Geometry: see drawing. Coordinates: mm, zero at the bounding-box minimum. A direction names the side the tool comes from. Give positions to 0.01 mm unless a question says otherwise; leave off trailing zeros. Order: outer loops, then holes, each group sorted by start corner. A loop starts at its lowest first (then second) coordinate and runs counter-clockwise, first axis right, second up. Notation, with made-up numbers: (20.25, 31) - (73.25, 31) arc R31 ccw to (73.25, 64) - close; hole circle Ø2 at (-13.75, 24). An arc over 180 degrees is marked (long way). One line per question, with ' | ' between items. Start each with the question number.
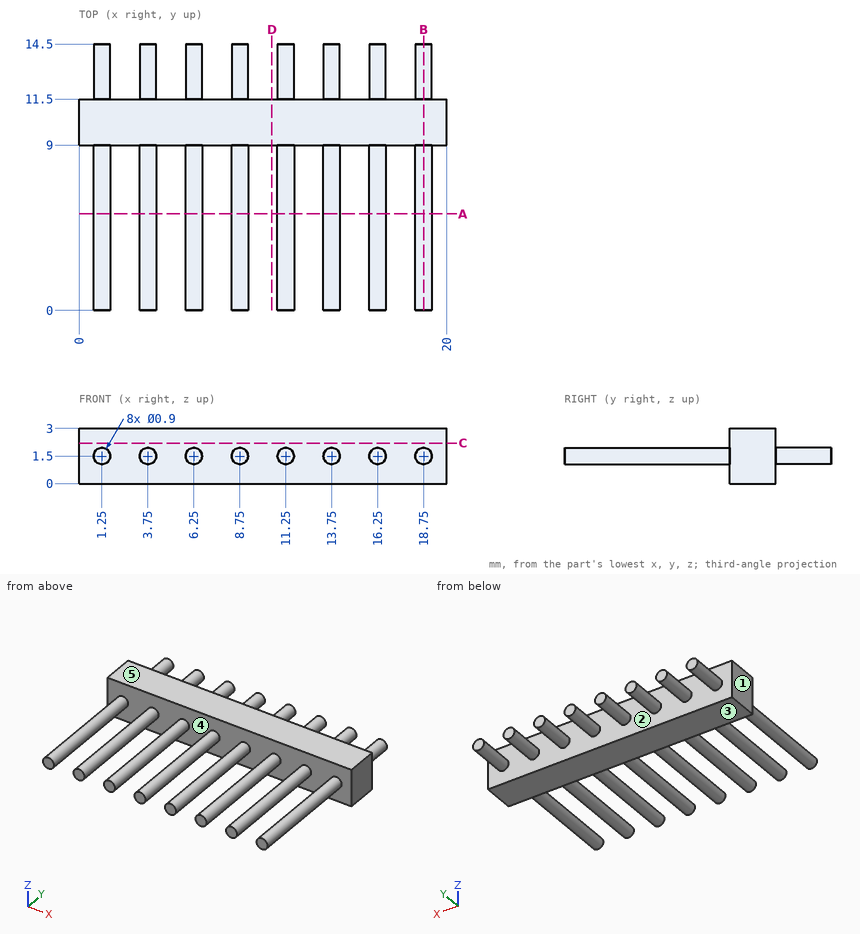
(1) Cut plane A-A, the plane y = 5.25. Return the cut outline in (x, z).
(2) Pull-direction query (X, two-part tool) for the marked faces 1, 2 and 3; classes: +X half, -X half, draft (parallel to the pull), parting line (faces both ways), or undercut.
(3) Cut plane B-B, the plane x = 18.75. Return the cut outline in (y, z).
(4) Material intervals for line 1 along Y through (x, z) = (14.75, 0.9); line 2 along Z through (x, y) = (13.5, 6.5), sorted ascending. Write a range as from..to.
(5) Cut plane C-C, the plane z = 2.2. Return the cut outline in (x, y), plus the area to 3 significant figures.
(6) Access query for the marked faces 4 and 5. Directions: +Z, -Z, +X, -X, +Y, -Y. A direction counts if a zero-diameter tool reaches every point of the face in a straight line with its end or side. Return the directions, or none.
(7) Cut plane D-D, the plane x = 10.5. Return the cut outline in (y, z).
Results are:
1) outline: circle Ø0.9 at (1.25, 1.5); circle Ø0.9 at (3.75, 1.5); circle Ø0.9 at (6.25, 1.5); circle Ø0.9 at (8.75, 1.5); circle Ø0.9 at (11.25, 1.5); circle Ø0.9 at (13.75, 1.5); circle Ø0.9 at (16.25, 1.5); circle Ø0.9 at (18.75, 1.5)
2) face 1: -X half | face 2: undercut | face 3: draft
3) outline: (0, 1.05) - (9, 1.05) - (9, 0) - (11.5, 0) - (11.5, 1.05) - (14.5, 1.05) - (14.5, 1.95) - (11.5, 1.95) - (11.5, 3) - (9, 3) - (9, 1.95) - (0, 1.95) - close
4) line 1: 9..11.5 | line 2: 1.13..1.87
5) outline: (0, 9) - (20, 9) - (20, 11.5) - (0, 11.5) - close | area: 50.0 mm2
6) face 4: -Y | face 5: +Z, +X, -X, +Y, -Y
7) outline: (9, 0) - (11.5, 0) - (11.5, 3) - (9, 3) - close
